Autodesk Inventor part; units mm, degrees
ref_plane "YZ Plane" through (0, 0, 0) normal (1, 0, 0) x (0, 1, 0)
ref_plane "XZ Plane" through (0, 0, 0) normal (0, 1, 0) x (-1, 0, 0)
ref_plane "XY Plane" through (0, 0, 0) normal (0, 0, 1) x (1, 0, 0)
sketch "Boceto1" plane through (0, 0, 0) normal (0, 0, 1) x (1, 0, 0)
  line L0 (-24.25, -22) -> (24.25, -22)
  line L1 (24.25, -22) -> (24.25, 22)
  line L2 (24.25, 22) -> (-24.25, 22)
  line L3 (-24.25, 22) -> (-24.25, -22)
  line L4 (-24.25, -22) -> (24.25, 22) construction
  line L5 (24.25, -22) -> (-24.25, 22) construction
  point P0 (0, 0)
  dimension "d0" = 48.5
  dimension "d1" = 44
extrude "Extrusión1" add sketch "Boceto1" along normal blind 48.5
sketch "Boceto2" plane through (-24.25, 22, 0) normal (0, 1, 0) x (1, 0, 0)
  line L0 (3, -3) -> (45.5, -3)
  line L1 (45.5, -3) -> (45.5, -45.5)
  line L2 (3, -45.5) -> (3, -3)
  line L3 (15.25, -45.5) -> (15.25, -48.5)
  line L4 (33.25, -45.5) -> (33.25, -48.5)
  line L5 (45.5, -45.5) -> (33.25, -45.5)
  line L6 (15.25, -45.5) -> (3, -45.5)
  line L7 (15.25, -48.5) -> (33.25, -48.5)
extrude "Extrusión2" cut sketch "Boceto2" against normal blind 40
sketch "Boceto5" plane through (-24.25, -22, 0) normal (0, -1, 0) x (1, 0, 0)
  line L0 (-10, 19.25) -> (0, 19.25)
  line L1 (0, 29.25) -> (-10, 29.25)
  line L2 (-10, 29.25) -> (-10, 19.25)
  line L3 (0, 0) -> (0, 48.5)
  line L4 (0, 19.25) -> (0, 29.25)
  line L5 (48.5, 19.25) -> (58.5, 19.25)
  line L6 (58.5, 19.25) -> (58.5, 29.25)
  line L7 (58.5, 29.25) -> (48.5, 29.25)
  line L8 (48.5, 0) -> (48.5, 48.5)
  line L9 (48.5, 19.25) -> (48.5, 29.25)
  circle A0 centre (53.5, 24.25) radius 2
  circle A1 centre (-5, 24.25) radius 2
  point P0 (24.25, 0)
  point P1 (0, 24.25)
  point P2 (48.5, 24.25)
  dimension "d15" = 4
  dimension "d16" = 4
extrude "Extrusión3" add sketch "Boceto5" against normal blind 3
properties part number "_3DPrint"
Check sheet for the modelled part. Datum: model origin and axes. Units: mm. A direction names the side the tool comes from. Round coordinates to 2 decimals unless told otherwise and drop trailing zeros. Order: outer loops, then holes, each group sorted by start corner. A loop starts at its lowest first (then second) coordinate and runs counter-clockwise, first axis right, second up.
(1) Go/stop test with flat-tipped pins: P1, Ø8, axis at y = 0.5, z = 30.5, coming from the +X side; P2, Ø1.5, axis at x = 31.5, y = -21, coming from the +Z side; P3, Ø12, axis at x = -20, y = -5, coming from the -Z side; P4, Ø11, axis at x = -30.5, z = 25, coming from the +Y side. Record where each tip stops, or that it passes through.
(2) Cross-section at A-A, the plane z = 24.25. Enter the section's corners in (x, y), and give its area (3 significant figures).
(3) Cross-section at D-D, the plane x = 17. Enter the section's corners in (y, z), and give its area (3 significant figures).
(4) Draft check along X on faces 4 (the flat face through (0, 0, 0)), 5 (the flat face through (21.25, 2, 24)), 6 (the flat face through (34.25, -21, 24)). Enter one of: pulls with the +X half, pulls with the -X half, needs draft (parallel to the pull), parting line crosses it, or undercut.
(5) Cross-section at B-B, the plane x = -29.25. Enter the section's corners in (y, z), and give its area (3 significant figures).
(6) Scan lines: probe 1 along X at (y, z) = (2, 20); probe 2 along Z at (x, y) = (12, -3); probe 3 along Y at (x, z) = (0.5, 26). Record each from-to range of solid material in increasing order.
(7) Access from +Z, -Z, +X, -X, +Y, -Y to the whole of each face (thin tool, end or side, straight path). Record for faces 1 (the flat face through (-29, -21, 29.25)), 2 (the flat face through (-9, 2, 47)), 3 (the flat face through (15, 2, 45.5)).
(8) Cross-section at C-C, the plane y = 12. Enter the section's corners in (x, z), and give its area (3 significant figures).
Check sheet entries:
1. P1: stops at x = 24.25
1. P2: stops at z = 29.25
1. P3: stops at z = 0
1. P4: stops at y = -19
2. outline: (-34.25, -22) - (-31.25, -22) - (-31.25, -19) - (-34.25, -19) - close; (-27.25, -22) - (27.25, -22) - (27.25, -19) - (24.25, -19) - (24.25, 22) - (21.25, 22) - (21.25, -18) - (-21.25, -18) - (-21.25, 22) - (-24.25, 22) - (-24.25, -19) - (-27.25, -19) - close; (31.25, -22) - (34.25, -22) - (34.25, -19) - (31.25, -19) - close
2. area: 470 mm2
3. outline: (-22, 0) - (22, 0) - (22, 3) - (-18, 3) - (-18, 45.5) - (22, 45.5) - (22, 48.5) - (-22, 48.5) - close
3. area: 434 mm2
4. face 4: needs draft
4. face 5: undercut
4. face 6: pulls with the +X half
5. outline: (-22, 19.25) - (-19, 19.25) - (-19, 22.25) - (-22, 22.25) - close; (-22, 26.25) - (-19, 26.25) - (-19, 29.25) - (-22, 29.25) - close
5. area: 18.0 mm2
6. probe 1: x = -24.25 to -21.25, 21.25 to 24.25
6. probe 2: z = 0 to 3, 45.5 to 48.5
6. probe 3: y = -22 to -18
7. face 1: +Z, -X, +Y, -Y
7. face 2: +Z, +Y
7. face 3: +Y
8. outline: (-24.25, 0) - (24.25, 0) - (24.25, 48.5) - (9, 48.5) - (9, 45.5) - (21.25, 45.5) - (21.25, 3) - (-21.25, 3) - (-21.25, 45.5) - (-9, 45.5) - (-9, 48.5) - (-24.25, 48.5) - close
8. area: 492 mm2
